from build123d import *

# Parameters (mm, degrees)
F0_W        = 35
F0_H        = 47
F1_DEPTH    = 2.5
F2_W        = 6
F2_H        = 1.5
F3_DEPTH    = 4
F4_W        = 15
F4_H        = 4
F5_DEPTH    = 2
F6_T1_DEPTH = 35
F7_W        = 11
F7_H        = 1
F8_DEPTH    = 1


# Not quite as in the source:
# - a fillet or chamfer that OpenCascade refuses, or shapes differently, is made with other operations: its cross-section is extruded or revolved along the edge and cut away or added


with BuildPart() as f1:
    # F0 (on Top) → F1 (new body)
    with BuildSketch(Plane.XY):
        with Locations((6.565169383, -0.3048535436)):
            Rectangle(F0_W, F0_H)
    extrude(amount=F1_DEPTH)

    # F2 (on face) → F3 (cut)
    with BuildSketch(Plane.XZ.offset(23.8048535436)):
        with Locations((-3.934830617, 0.75)):
            Rectangle(F2_W, F2_H)
        with Locations((17.065169383, 0.75)):
            Rectangle(F2_W, F2_H)
    extrude(amount=-F3_DEPTH, mode=Mode.SUBTRACT)

    # F4 (on face) → F5 (join)
    with BuildSketch(Plane(origin=(0, 0, 0), x_dir=(1, 0, 0), z_dir=(0, 0, -1))):
        with Locations((6.565169383, -21.1951464564)):
            Rectangle(F4_W, F4_H)
    extrude(amount=F5_DEPTH)

    # F6: fillet of radius 5 on 1 edges, made by hand

    # F6_s2 → F6_t1 (cut)
    with BuildSketch(Plane.YZ.offset(-10.934830617)):
        with BuildLine():
            ThreePointArc((19.1951464564, 0), (20.9590784789, -1.472135955), (23.1951464564, -2))
            Line((23.1951464564, -2), (19.1951464564, -2))
            Line((19.1951464564, -2), (19.1951464564, 0))
        make_face()
    extrude(amount=F6_T1_DEPTH, mode=Mode.SUBTRACT)

    # F7 (on face) → F8 (cut)
    with BuildSketch(Plane(origin=(0, 23.1951464564, 0), x_dir=(-1, 0, 0), z_dir=(0, 1, 0))):
        with Locations((-6.565169383, -1)):
            Rectangle(F7_W, F7_H)
    extrude(amount=-F8_DEPTH, mode=Mode.SUBTRACT)


solid = f1.part
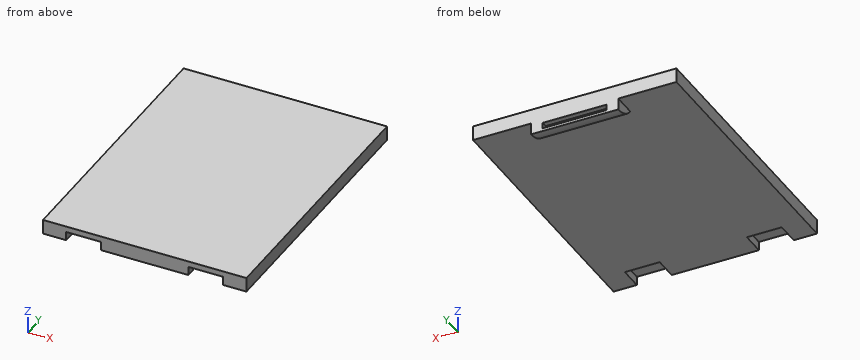
Source: CAD feature listing. Evaluate the final solid. Frame: model axes, mm. Give positions to 0.01 mm unless a question says otherwise; leave off trailing zeros. Order: outer loops, then holes, each group sorted by start corner. A loop starts at its lowest first (then second) coordinate and runs counter-clockwise, first axis right, second up. Notation, with made-up numbers: (48, -8) -> (93, -8) arc R13 cw to (93, 15) -> close; hole circle Ø5 at (2.5, -22). An arc over 180 degrees is marked (long way). Write item = value, one per line.
Q1. Pin query (flat end, axial travel): pin 1 (1.6 mm diameter, centred on y = 21, z = -1, fed in from +X); pin 2 (2 mm diameter, centred on x = 16.5, y = -21, fed in from -Z); pin 3 (8 mm diameter, centred on x = -4, y = -2.5, fed in from -Z). Return the tip coordinate at first contact, or that it passes through.
Data:
pin_1 = 14.07
pin_2 = 1.5
pin_3 = 0
Q2. Cut plane B-B, the plane y = -13. Output: boundary loops of the cut face in (x, z), and give its area (3 significant figures).
Data:
outline = (-10.93, 0) -> (24.07, 0) -> (24.07, 2.5) -> (-10.93, 2.5) -> close
area = 87.5 mm^2
Q3. Cut plane A-A, the plane x = 7. Output: boundary loops of the cut face in (y, z).
Data:
outline = (-23.8, 0) -> (19.2, 0) arc R5 ccw to (23.2, -2) -> (23.2, -1.5) -> (22.2, -1.5) -> (22.2, -0.5) -> (23.2, -0.5) -> (23.2, 2.5) -> (-23.8, 2.5) -> close
Q4. Cut plane C-C, the plane x = 13.5. Output: boundary loops of the cut face in (y, z), and give its area (3 significant figures).
Data:
outline = (-23.8, 0) -> (19.2, 0) arc R5 ccw to (23.2, -2) -> (23.2, 2.5) -> (-23.8, 2.5) -> close
area = 123 mm^2
Q5. Material intervals for line 1 (X direction, y = -20, z = 0.35); line 2 (Z direction, x = 14.5, y = 11.5); line 3 (Z direction, x = -3, y = -22), sorted ascending. Write a range as from..to.
Data:
line_1 = -10.93..-6.93, -0.93..14.07, 20.07..24.07
line_2 = 0..2.5
line_3 = 1.5..2.5
Q6. Cut plane D-D, the plane x = -9. Output: boundary loops of the cut face in (y, z), and give its area (4 significant figures).
Data:
outline = (-23.8, 0) -> (23.2, 0) -> (23.2, 2.5) -> (-23.8, 2.5) -> close
area = 117.5 mm^2
